Could you check a few things on this model? Use its own coordinates, in mm. Face numbers are marked on the shaded views. A direction names the side the tool comes from. Round coordinates to 2 decimals unless told otherwise and drop trailing zeros. Write each loop counter-clockwise with the first axis right and the second up, starting at its lowest first coordinate (ties: lowest second). Pieces come first, ordered by that corner, then holes. Notation, with made-up numbers: (38.25, -19) - (79.25, -19) arc R18 cw to (79.25, 1) - close; hole circle Ø11 at (66, -5.5). An arc over 180 degrees is marked (long way). Put each result on its own line as item: value.
from build123d import *

# Parameters (mm, degrees)
F0_W     = 38.1
F0_H     = 31.75
F1_DEPTH = 25.4
F3_DEPTH = 50.8


with BuildPart() as f1:
    # F0 (on Front) → F1 (new body)
    with BuildSketch(Plane.XZ):
        with Locations((19.05, 15.875)):
            Rectangle(F0_W, F0_H)
    extrude(amount=F1_DEPTH)

    # F2 (on face) → F3 (cut)
    with BuildSketch(Plane.YZ.offset(38.1)):
        Polygon((0, 31.75), (-12.7, 31.75), (-6.35, 12.7), (0, 12.7), align=None)
    extrude(amount=-F3_DEPTH, mode=Mode.SUBTRACT)


solid = f1.part
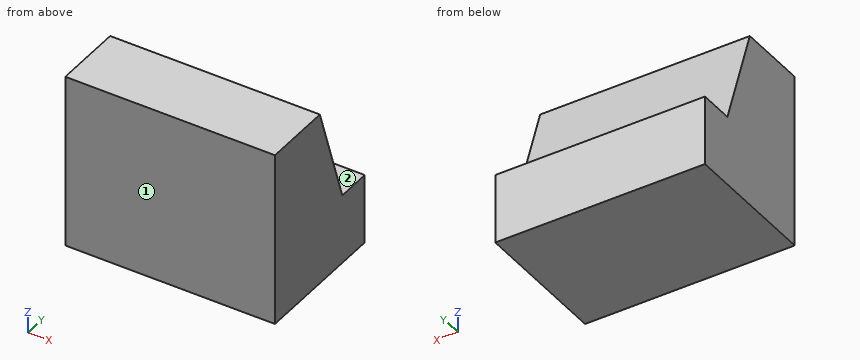
(1) For the marked faces 1 and 2, which set-ups out of +Z, -Z, +X, -X, +Y, -Y let a thin tool reach every point of the face, with its end or its side?
Values found:
face 1: +Z, -Z, +X, -X, -Y
face 2: +Z, +X, -X, +Y
(2) Imagine slicing it at A-A, the plane x = 6.5. List the corners of the cut face in (y, z) for me, then the cut area to 3 significant figures.
Values found:
outline: (-25.4, 0) - (0, 0) - (0, 12.7) - (-6.35, 12.7) - (-12.7, 31.75) - (-25.4, 31.75) - close
area: 625 mm^2
(3) Imagine slicing it at B-B, the plane z = 28. List the corners of the cut face in (x, y) for me, then the cut area to 3 significant figures.
Values found:
outline: (0, -25.4) - (38.1, -25.4) - (38.1, -11.45) - (0, -11.45) - close
area: 531 mm^2
(4) I'm going to push a flat-ended pin straight in: pin 1 (5 mm diameter, centred on x = 24.5, y = -3, fed in from +Z). Where does the tip first touch, or does it pass through?
Values found:
pin 1: stops at z = 12.7
(5) Please list where these lines run through material, in increasing order: probe 1 along Z at (x, y) = (20, -4); probe 2 along Y at (x, z) = (3, 21); probe 3 along Y at (x, z) = (25, 14.5). Write a range as from..to.
Values found:
probe 1: z = 0..12.7
probe 2: y = -25.4..-9.12
probe 3: y = -25.4..-6.95
(6) Imagine slicing it at C-C, the plane y = -8.25. List the corners of the cut face in (x, z) for me, then the cut area to 3 significant figures.
Values found:
outline: (0, 0) - (38.1, 0) - (38.1, 18.4) - (0, 18.4) - close
area: 701 mm^2
